```python
from build123d import *

# Parameters (mm, degrees)
F0_W          = 43.4
F0_H          = 38
F0_R          = 3
F1_DEPTH      = 2
F2_R          = 12.55
F2_R_2        = 10.9
F3_DEPTH      = 21.7
F3_DEPTH_BACK = 21.7
F4_R          = 5
F5_DEPTH      = 27.151
F8_R          = 10


# Not quite as in the source:
# - a feature names something its author has since deleted; it is built from what else it names


with BuildPart() as f1:
    # F0 (on Front) → F1 (new body)
    with BuildSketch(Plane.XZ):
        with Locations((0, -1)):
            Rectangle(F0_W, F0_H)
        Circle(F0_R, mode=Mode.SUBTRACT)
    extrude(amount=F1_DEPTH)

    # F2 (on Right) → F3 (join, two sides)
    with BuildSketch(Plane.YZ) as f3_sk:
        with BuildLine():
            ThreePointArc((-27.0737723252, 12.9281979258), (-25.4648034923, 7.5886797024), (-26.9655996144, 2.217753659))
            ThreePointArc((-26.9655996144, 2.217753659), (-28.5932479144, -1.4635839649), (-29.15, -5.45))
            Line((-29.15, -5.45), (-29.15, -20))
            Line((-29.15, -20), (-2, -20))
            Line((-2, -20), (-2, 18))
            Line((-2, 18), (0, 18))
            Line((0, 18), (-5.2100705327, 26.6195334989))
            ThreePointArc((-5.2100705327, 26.6195334989), (-23.0965208991, 30.8796696778), (-27.0737723252, 12.9281979258))
        make_face()
        with Locations((-14.6, -5.45)):
            Circle(F2_R, mode=Mode.SUBTRACT)
        with Locations((-16.25, 19.9464564457)):
            Circle(F2_R_2, mode=Mode.SUBTRACT)
    extrude(amount=-F3_DEPTH)
    extrude(f3_sk.sketch, amount=F3_DEPTH_BACK)

    # F4 (on face) → F5 (cut, through all)
    with BuildSketch(Plane(origin=(0, -2, 0), x_dir=(-1, 0, 0), z_dir=(0, 1, 0))):
        Circle(F4_R)
    extrude(amount=-F5_DEPTH, mode=Mode.SUBTRACT)

    # F6 (on Top) → F7 (revolve, cut)
    with BuildSketch(Plane.XY):
        Polygon((0, -2), (0, 0), (-3, 0), (-3, -0.3), (-5, -2), align=None)
    revolve(axis=Axis((0, -1, 0), (0, -1, 0)), mode=Mode.SUBTRACT)

    # F8
    f8_edges = [f1.edges().sort_by_distance(p)[0] for p in [
        (0, 0, -20),
        (0, 0, 18),
        (0, -29.15, -20),
    ]]
    fillet(f8_edges, radius=F8_R)


solid = f1.part
```
Here's how the part is built. I have some questions about the finished solid (model axes, mm). A direction names the side the tool comes from. Round coordinates to 2 decimals unless told otherwise and drop trailing zeros. Write each loop counter-clockwise with the first axis right and the second up, starting at its lowest first coordinate (ties: lowest second). Pieces come first, ordered by that corner, then holes.
Q1. If we mould it in two halves opening along Z, with no side actions, what happens to faces 4 (the cylindrical face through (-0.304, -24.284, 27.313)), 5 (the flat face through (-0.3, -3.3, 23.46)), 6 (the flat face through (-21.7, -9, 7))? For each: +Z half, -Z half, draft (parallel to the pull), parting line (faces both ways), or undercut.
Q2. If we section it at B-B on x = 0: Write out the boundary of the cut face in (y, z).
Q3. If we section it at A-A on y = -14.6: Write out the boundary of the cut face in (x, z), plus the area to 3 significant figures.
Q4. If we section it at D-D on z = 24: Write out the boundary of the cut face in (x, y), plus the area to 3 significant figures.
Q5. Please list where these lines run through material, in increasing order: probe 1 along Z at (x, y) = (9, -19.75); probe 2 along Z at (x, y) = (6, -16.25); probe 3 along Z at (x, y) = (-5, -4.75).
Q6. If we section it at C-C on z = 0: Write out the boundary of the cut face in (x, y).
Q7. Will these pins go through, and if not, where does the flat tip stop? P1, Ø1.5, axis at x = -6.5, y = -14.5, coming from the +Z side; P2, Ø1.5, axis at x = 7, y = -21.5, coming from the -Z side; P3, Ø3, axis at x = 6.5, y = -4.5, coming from the +Z side; P4, Ø3.5, axis at x = 0, z = 0, coming from the -Y side.
Q8. Which directions (+Z, -Z, +X, -X, +Y, -Y) give clear straight access to the entire face, cutting with the end or side of a thin tool? Please do faces 1 (the cylindrical face through (-5.126, -28.578, -1.409)), 2 (the flat face through (21.7, -9, 7)), 3 (the cylindrical face through (0, -4, 5)).
Answer below:
1. face 4: undercut
1. face 5: +Z half
1. face 6: draft
2. outline: (-29.15, -10) arc R10 ccw to (-19.15, -20) - (-10, -20) arc R10 ccw to (0, -10) - (0, -3) - (-0.3, -3) - (-2, -5) - (-2.06, -5) arc R12.55 cw (long way) to (-27.14, -5) - (-29.14, -5) arc R14.55 ccw to (-29.15, -5.45) - close; (-27.07, 12.93) arc R10 cw to (-25.78, 5) - (-21.55, 5) arc R12.55 cw to (-7.65, 5) - (-2, 5) - (-0.3, 3) - (0, 3) - (0, 15.21) arc R10 ccw to (-1.44, 20.39) - (-5.21, 26.62) arc R12.9 ccw (long way) to start; hole circle Ø21.8 at (-16.25, 19.95)
3. outline: (-21.7, -20) - (21.7, -20) - (21.7, -18) - (-21.7, -18) - close; (-21.7, 7.1) - (21.7, 7.1) - (21.7, 9.17) - (-21.7, 9.17) - close; (-21.7, 30.72) - (21.7, 30.72) - (21.7, 32.74) - (-21.7, 32.74) - close
3. area: 264 mm2
4. outline: (-21.7, -28.5) - (21.7, -28.5) - (21.7, -26.37) - (-21.7, -26.37) - close; (-21.7, -6.13) - (21.7, -6.13) - (21.7, -3.63) - (-21.7, -3.63) - close
4. area: 201 mm2
5. probe 1: z = -19.98 to -16.89, 5.99 to 9.62, 30.27 to 32.36
5. probe 2: z = -20 to -17.89, 6.99 to 9.05, 30.85 to 32.85
5. probe 3: z = -18.51 to -13.23, 2.33 to 25.86
6. outline: (-21.7, -28.09) - (-5, -28.09) - (-5, -25.9) - (-21.7, -25.9) - close; (-21.7, -3.3) - (-5, -3.3) - (-5, -2) - (-3, -0.3) - (-3, 0) - (-21.7, 0) - close; (3, -0.3) - (5, -2) - (5, -3.3) - (21.7, -3.3) - (21.7, 0) - (3, 0) - close; (5, -28.09) - (21.7, -28.09) - (21.7, -25.9) - (5, -25.9) - close
7. P1: stops at z = 32.81
7. P2: stops at z = -19.87
7. P3: stops at z = 27.78
7. P4: passes through
8. face 1: +X, -X, -Y
8. face 2: +Z, -Z, +X, +Y, -Y
8. face 3: -Y
